from build123d import *

# Parameters (mm, degrees)
SKETCH_1_R          = 2.1
SKETCH_1_R_2        = 10.5
SKETCH_1_R_3        = 10
EXTRUDE_1_DEPTH     = 4
CHAMFER_1_SIZE      = 5
FILLET_1_R          = 10
SKETCH_2_R          = 2.1
CUT_EXTRUDE_1_DEPTH = 10
EXTRUDE_START       = -4
SKETCH_3_R          = 1.6
EXTRUDE_2_DEPTH     = 4
FILLET_2_R          = 3
FILLET_3_R          = 11
SKETCH_4_R          = 1.6
EXTRUDE_3_DEPTH     = 4
FILLET_4_R          = 10
CHAMFER_2_SIZE      = 2
CHAMFER_2_SIZE2     = 1.851556395
FILLET_5_R          = 10
SKETCH_5_R          = 17.5
CUT_EXTRUDE_2_DEPTH = 10


with BuildPart() as part:
    # 草图1 → 凸台-拉伸1 (new body)
    with BuildSketch(Plane(origin=(0, 0, 0), x_dir=(1, 0, 0), z_dir=(0, 1, 0))):
        Polygon((0, 31.819805153), (-31.819805153, 0), (0, -31.819805153), (15.909902577, -15.909902577), (67.5, -15.909902577), (67.5, -22.5), (112.5, -22.5), (112.5, 22.5), (67.5, 22.5), (67.5, 15.909902577), (15.909902577, 15.909902577), align=None)
        with Locations(Location((0, 14, 0), (0, 0, 270))):
            Circle(SKETCH_1_R, mode=Mode.SUBTRACT)
        with Locations(Location((14, 0, 0), (0, 0, 270))):
            Circle(SKETCH_1_R, mode=Mode.SUBTRACT)
        with Locations(Location((0, -14, 0), (0, 0, 270))):
            Circle(SKETCH_1_R, mode=Mode.SUBTRACT)
        with Locations(Location((-14, 0, 0), (0, 0, 270))):
            Circle(SKETCH_1_R, mode=Mode.SUBTRACT)
        with Locations(Location((90, 0, 0), (0, 0, 270))):
            Circle(SKETCH_1_R_2, mode=Mode.SUBTRACT)
        with Locations(Location((0, 22.5, 0), (0, 0, 270))):
            Circle(SKETCH_1_R, mode=Mode.SUBTRACT)
        with Locations(Location((0, -22.5, 0), (0, 0, 270))):
            Circle(SKETCH_1_R, mode=Mode.SUBTRACT)
        with Locations(Location((0, 0, 0), (0, 0, 270))):
            Circle(SKETCH_1_R_3, mode=Mode.SUBTRACT)
        with Locations(Location((-22.5, 0, 0), (0, 0, 270))):
            Circle(SKETCH_1_R, mode=Mode.SUBTRACT)
    extrude(amount=EXTRUDE_1_DEPTH)

    # 倒角1
    chamfer_1_edges = [part.edges().sort_by_distance(p)[0] for p in [
        (112.5, 2, -22.5),
        (112.5, 2, 22.5),
        (0, 2, 31.819805153),
        (-31.819805153, 2, 0),
        (0, 2, -31.819805153),
    ]]
    chamfer(chamfer_1_edges, length=CHAMFER_1_SIZE)

    # 圆角1
    # the kernel refuses this fillet: 10 mm, written as the material it adds along each edge
    with BuildSketch(Plane(origin=(15.909902577, 0, -15.909902577), x_dir=(-0.707106781186552, 0, -0.707106781186543), z_dir=(0, 1, 0))) as fillet_1_piece_1:
        with BuildLine():
            CenterArc((FILLET_1_R * 0.414213562373, -FILLET_1_R), FILLET_1_R, 90, 45)
            Line((-FILLET_1_R * 0.292893218813, -FILLET_1_R * 0.292893218813), (-FILLET_1_R * 0.307035354437, -FILLET_1_R * 0.27875108319))
            Line((-FILLET_1_R * 0.307035354437, -FILLET_1_R * 0.27875108319), (-FILLET_1_R * 0.00828427124746, FILLET_1_R * 0.02))
            Line((-FILLET_1_R * 0.00828427124746, FILLET_1_R * 0.02), (FILLET_1_R * 0.414213562373, FILLET_1_R * 0.02))
            Line((FILLET_1_R * 0.414213562373, FILLET_1_R * 0.02), (FILLET_1_R * 0.414213562373, 0))
        make_face()
    extrude(amount=4)
    with BuildSketch(Plane(origin=(15.909902577, 0, 15.909902577), x_dir=(-0.7071067811865422, 0, 0.707106781186553), z_dir=(0, 1, 0))) as fillet_1_piece_2:
        with BuildLine():
            CenterArc((FILLET_1_R * 0.414213562373, FILLET_1_R), FILLET_1_R, 225, 45)
            Line((-FILLET_1_R * 0.292893218813, FILLET_1_R * 0.292893218813), (-FILLET_1_R * 0.307035354437, FILLET_1_R * 0.27875108319))
            Line((-FILLET_1_R * 0.307035354437, FILLET_1_R * 0.27875108319), (-FILLET_1_R * 0.00828427124746, -FILLET_1_R * 0.02))
            Line((-FILLET_1_R * 0.00828427124746, -FILLET_1_R * 0.02), (FILLET_1_R * 0.414213562373, -FILLET_1_R * 0.02))
            Line((FILLET_1_R * 0.414213562373, -FILLET_1_R * 0.02), (FILLET_1_R * 0.414213562373, 0))
        make_face()
    extrude(amount=4)
    with BuildSketch(Plane(origin=(67.5, 0, 15.909902577), x_dir=(-1, 0, 0), z_dir=(0, 1, 0))) as fillet_1_piece_3:
        with BuildLine():
            CenterArc((9.400668296, 10), FILLET_1_R, 199.937217397, 70.062782603)
            Line((0, 6.590097423), (-0.188013366, 6.521899372))
            ThreePointArc((-0.188013366, 6.521899372), (-0.2, 3.295048712), (-0.2, 0))
            Line((-0.2, 0), (0, -0.2))
            Line((0, -0.2), (9.400668296, -0.2))
            Line((9.400668296, -0.2), (9.400668296, 0))
        make_face()
    extrude(amount=4)
    with BuildSketch(Plane(origin=(67.5, 0, -15.909902577), x_dir=(-1, 0, 0), z_dir=(0, 1, 0))) as fillet_1_piece_4:
        with BuildLine():
            CenterArc((9.400668296, -10), FILLET_1_R, 90, 70.062782603)
            Line((0, -6.590097423), (-0.188013366, -6.521899372))
            ThreePointArc((-0.188013366, -6.521899372), (-0.2, -3.295048712), (-0.2, 0))
            Line((-0.2, 0), (0, 0.2))
            Line((0, 0.2), (9.400668296, 0.2))
            Line((9.400668296, 0.2), (9.400668296, 0))
        make_face()
    extrude(amount=4)

    # 草图2 → 切除-拉伸1 (cut)
    with BuildSketch(Plane.XZ):
        with Locations(Location((106.464466094, 16.464466094, 0), (0, 0, 270))):
            Circle(SKETCH_2_R)
        with Locations(Location((106.464466094, -16.464466094, 0), (0, 0, 270))):
            Circle(SKETCH_2_R)
        with Locations(Location((73.535533906, -16.464466094, 0), (0, 0, 90))):
            Circle(SKETCH_2_R)
        with Locations(Location((73.535533906, 16.464466094, 0), (0, 0, 90))):
            Circle(SKETCH_2_R)
        with Locations(Location((24.075684952, 10.909902577, 0), (0, 0, 270))):
            Circle(SKETCH_2_R)
        with Locations(Location((59.075684952, 10.909902577, 0), (0, 0, 270))):
            Circle(SKETCH_2_R)
        with Locations(Location((59.075684952, -10.909902577, 0), (0, 0, 90))):
            Circle(SKETCH_2_R)
        with Locations(Location((24.075684952, -10.909902577, 0), (0, 0, 90))):
            Circle(SKETCH_2_R)
    extrude(amount=-CUT_EXTRUDE_1_DEPTH, mode=Mode.SUBTRACT)

    # 草图3 → 凸台-拉伸2 (add)
    with BuildSketch(Plane(origin=(0, 4, 0), x_dir=(1, 0, 0), z_dir=(0, 1, 0)).offset(EXTRUDE_START)):
        with BuildLine():
            Line((3.535533906, 28.284271247), (40.057636417, 81.344203773))
            ThreePointArc((40.057636417, 81.344203773), (45.94930127, 83.86671265), (50.75784592, 79.629654221))
            Line((50.75784592, 79.629654221), (67.5, 22.5))
            ThreePointArc((67.5, 22.5), (63.839583189, 17.721525883), (58.099331704, 15.909902577))
            Line((58.099331704, 15.909902577), (20.0520382, 15.909902577))
            ThreePointArc((20.0520382, 15.909902577), (16.225203877, 16.671107252), (12.980970389, 18.838834765))
            Line((12.980970389, 18.838834765), (3.535533906, 28.284271247))
        make_face()
        with Locations(Location((45, 77.942286341, 0), (0, 0, 270))):
            Circle(SKETCH_3_R, mode=Mode.SUBTRACT)
        Polygon((16.491758356, 29.470182421), (43.526560522, 68.746803428), (56.080145943, 25.909902577), (20.0520382, 25.909902577), align=None, mode=Mode.SUBTRACT)
    extrude(amount=EXTRUDE_2_DEPTH)

    # 圆角2
    fillet_2_edges = [part.edges().sort_by_distance(p)[0] for p in [
        (16.491758356, 2, -29.470182421),
        (43.526560522, 2, -68.746803428),
        (56.080145943, 2, -25.909902577),
        (20.0520382, 2, -25.909902577),
    ]]
    fillet(fillet_2_edges, radius=FILLET_2_R)

    # 圆角3
    fillet_3_edges = [part.edges().sort_by_distance(p)[0] for p in [
        (67.5, 2, -22.5),
        (3.535533906, 2, -28.284271247),
    ]]
    fillet(fillet_3_edges, radius=FILLET_3_R)

    # 草图4 → 凸台-拉伸3 (add)
    with BuildSketch(Plane(origin=(0, 4, 0), x_dir=(1, 0, 0), z_dir=(0, 1, 0)).offset(EXTRUDE_START)):
        with BuildLine():
            Line((45.94930127, 83.86671265), (81.347717681, 83.86671265))
            Line((81.347717681, 83.86671265), (107.5, 22.5))
            Line((107.5, 22.5), (97.716806526, 22.5))
            Line((97.716806526, 22.5), (75.4, 74.86671265))
            Line((75.4, 74.86671265), (52.153651701, 74.86671265))
            Line((52.153651701, 74.86671265), (50.75784592, 79.629654221))
            ThreePointArc((50.75784592, 79.629654221), (48.966689034, 82.443994695), (45.94930127, 83.86671265))
        make_face()
        with Locations(Location((78, 77.942286341, 0), (0, 0, 270))):
            Circle(SKETCH_4_R, mode=Mode.SUBTRACT)
    extrude(amount=EXTRUDE_3_DEPTH)

    # 圆角4
    fillet_4_edges = [part.edges().sort_by_distance(p)[0] for p in [
        (97.716806526, 2, -22.5),
        (75.4, 2, -74.86671265),
        (52.153651701, 2, -74.86671265),
    ]]
    fillet(fillet_4_edges, radius=FILLET_4_R)

    # 倒角2
    chamfer_2_edges = [part.edges().sort_by_distance(p)[0] for p in [
        (81.347717681, 2, -83.86671265),
    ]]
    chamfer_2_side = [part.faces().sort_by_distance(p)[0] for p in [
        (63.648509476, 2, -83.86671265),
    ]]
    chamfer(chamfer_2_edges, length=CHAMFER_2_SIZE, length2=CHAMFER_2_SIZE2, reference=chamfer_2_side[0])

    # 圆角5
    fillet_5_edges = [part.edges().sort_by_distance(p)[0] for p in [
        (107.5, 2, -22.5),
    ]]
    fillet(fillet_5_edges, radius=FILLET_5_R)

    # 草图5 → 切除-拉伸2 (cut)
    with BuildSketch(Plane(origin=(0, 4, 0), x_dir=(1, 0, 0), z_dir=(0, 1, 0))):
        with Locations(Location((0, 0, 0), (0, 0, 270))):
            Circle(SKETCH_5_R)
    extrude(amount=-CUT_EXTRUDE_2_DEPTH, mode=Mode.SUBTRACT)


solid = part.part
Part model, mm, in its own coordinate system. A direction names the side the tool comes from. Round coordinates to 2 decimals unless told otherwise and drop trailing zeros. Loops run counter-clockwise (first coordinate to the right, second up) from the corner with the lowest first, then second, coordinate; pieces in that order, holes last. Notation, with made-up numbers: (51, 69) - (102, 69) arc R30 ccw to (102, 105) - close; hole circle Ø11 at (-39, 58.5). An arc over 180 degrees is marked (long way). Answer as a JSON object with one key per item and string values.
Item 1: Band-saw the part on C-C on z = -50.5. List the corners of the cut face in (x, y).
Output:
{"outline": "(18.83, 0) - (30.97, 0) - (30.97, 4) - (18.83, 4) - close; (48.87, 0) - (59.29, 0) - (59.29, 4) - (48.87, 4) - close; (85.78, 0) - (95.57, 0) - (95.57, 4) - (85.78, 4) - close"}
Item 2: Pull direction Z, two halves, no side cores. Call faces 1 (the face through (-0.8, 1.97, 24.44)), 2 (the face through (62, 2, -83.867)), 3 (the face through (87, 2, 22.5)): pulls with the +Z half, pulls with the -Z half, needs draft (parallel to the pull), parting line crosses it, or undercut.
Output:
{"face 1": "undercut", "face 2": "pulls with the -Z half", "face 3": "pulls with the +Z half"}
Item 3: Pin check, flat tips, straight feed: pin 1 (1.6 mm diameter, centred on x = 67, y = 1.5, fed in from +Z); pin 2 (2 mm diameter, centred on y = 2, z = -55.5, fed in from +X). Stop position of each tip, or through.
Output:
{"pin 1": "z = 22.5", "pin 2": "x = 93.86"}
Item 4: Wall check: L1, parallel to X at y = 2.4, z = 0; L2, parallel to Z at x = 78, y = 3.7; L3, parallel to X at y = 1.3, z = -47.5. Give the ranges that are in metal, low to high.
Output:
{"L1": "-28.28 to -24.6, -20.4 to -17.5, 17.5 to 79.5, 100.5 to 112.5", "L2": "-83.87 to -79.54, -76.34 to -68.77, -22.5 to 22.5", "L3": "16.76 to 28.9, 49.75 to 60.17, 87.06 to 96.85"}
Item 5: Band-saw the part on B-B on x = -22.5. List the corners of the cut face in (y, z).
Output:
{"outline": "(0, -9.32) - (4, -9.32) - (4, -2.1) - (0, -2.1) - close; (0, 2.1) - (4, 2.1) - (4, 9.32) - (0, 9.32) - close"}
Item 6: Band-saw the part on A-A on z = 0. List the corners of the cut face in (x, y), plus the area to 3 significant figures.
Output:
{"outline": "(-28.28, 0) - (-24.6, 0) - (-24.6, 4) - (-28.28, 4) - close; (-20.4, 0) - (-17.5, 0) - (-17.5, 4) - (-20.4, 4) - close; (17.5, 0) - (79.5, 0) - (79.5, 4) - (17.5, 4) - close; (100.5, 0) - (112.5, 0) - (112.5, 4) - (100.5, 4) - close", "area": "322 mm2"}
Item 7: Band-saw the part on D-D on x = 0. List the corners of the cut face in (y, z), plus the area to 3 significant figures.
Output:
{"outline": "(0, -28.52) - (4, -28.52) - (4, -24.6) - (0, -24.6) - close; (0, -20.4) - (4, -20.4) - (4, -17.5) - (0, -17.5) - close; (0, 17.5) - (4, 17.5) - (4, 20.4) - (0, 20.4) - close; (0, 24.6) - (4, 24.6) - (4, 28.28) - (0, 28.28) - close", "area": "53.6 mm2"}
Item 8: Tool access for faces 4 (the face through (16.28, 1.97, 16.65)), 5 (the face through (94.235, 1.972, -53.628)), 6 (the face through (50.06, 1.97, -46.45)): list every direction of +Z, -Z, +X, -X, +Y, -Y with a clear straight run to the whole face (end or side of a thin tool).
Output:
{"face 4": "+Z, +Y, -Y", "face 5": "-Z, +X, +Y, -Y", "face 6": "+Y, -Y"}
